from build123d import *

# Parameters (mm, degrees)
F1_DEPTH = 430
F3_DEPTH = 60.001
F4_R     = 4.5
F5_DEPTH = 60.001


with BuildPart() as f1:
    # F0 (on Front) → F1 (new body)
    with BuildSketch(Plane.XZ):
        Polygon((60, 0), (0, 0), (0, -60), (2.5, -60), (2.5, -2.5), (60, -2.5), align=None)
    extrude(amount=F1_DEPTH)

    # F2 (on face) → F3 (cut, through all)
    with BuildSketch(Plane(origin=(0, 0, 0), x_dir=(0, -1, 0), z_dir=(-1, 0, 0))):
        Polygon((0, 0), (0, -60), (60, -60), align=None)
        Polygon((370, -60), (430, -60), (430, 0), align=None)
    extrude(amount=-F3_DEPTH, mode=Mode.SUBTRACT)

    # F4 (on face) → F5 (cut, through all)
    with BuildSketch(Plane.XY):
        with Locations((30, -90)):
            Circle(F4_R)
        with Locations((30, -190)):
            Circle(F4_R)
        with Locations((30, -330)):
            Circle(F4_R)
        with Locations((30, -400)):
            Circle(F4_R)
    extrude(amount=-F5_DEPTH, mode=Mode.SUBTRACT)


solid = f1.part
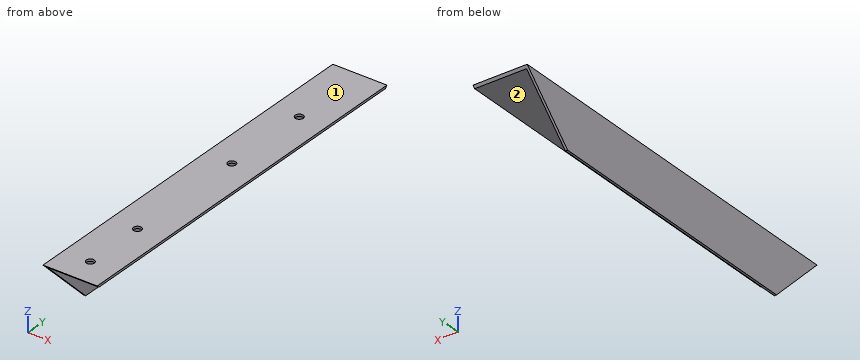
Here's how the part is built. I have some questions about the finished solid (model axes, mm). Face numbers are marked on the shaded views. A direction names the side the tool comes from. Round coordinates to 2 decimals unless told otherwise and drop trailing zeros. Loops run counter-clockwise (first coordinate to the right, second up) from the corner with the lowest first, then second, coordinate; pieces in that order, holes last. Notation, with made-up numbers: M 48.25,-25.75 L 72.25,-25.75 A27 cw 72.25,-1.75 Z; hole C 79.5,-7.5 d3. An arc over 180 degrees is marked long. Write each question's results on one line, items separated by ' | '. Start each with the question number.
(1) I want a section at A-A (y = -330). Please give me the cut outline in (x, z).
(2) On a 3-axis mill with a long thin cutter (end or side, diameter ignored), from which of +Z, -Z, +X, -X, +Y, -Y can I reach the whole of each face in a straight line? I mean the marked faces 1 and 2. Say none if no direction works.
(3) I want a section at C-C (y = -400). Please give me the cut outline in (x, z), then the cut area to 3 significant figures.
(4) I want a section at B-B (x = 30). Please give me the cut outline in (y, z).
(5) If I drill on probe 1 along X at (y, z) = (-330, -1.75); probe 2 along Y at (x, z) = (30, -1.9); probe 3 along Y at (x, z) = (30, -1.45), over which ranges is the centre line in solid material (lowest first)? Write a range as from..to.
(6) Will these pins go through, and if not, where does the flat tip stop? P1, Ø17.5, axis at y = -248, z = -25.5, coming from the +X side; P2, Ø5, axis at x = 8, y = -204, coming from the -Z side.
(7) I want a section at D-D (z = -47.5). Please give me the cut outline in (x, y).
Solved:
1) outline: M 0,-60 L 2.5,-60 L 2.5,-2.5 L 25.5,-2.5 L 25.5,0 L 0,0 Z; M 34.5,-2.5 L 60,-2.5 L 60,0 L 34.5,0 Z
2) face 1: +Z, +X, -X, +Y, -Y | face 2: -Z, +X, +Y, -Y
3) outline: M 0,-30 L 2.5,-30 L 2.5,-2.5 L 25.5,-2.5 L 25.5,0 L 0,0 Z; M 34.5,-2.5 L 60,-2.5 L 60,0 L 34.5,0 Z | area: 196 mm²
4) outline: M -430,0 L -427.5,-2.5 L -404.5,-2.5 L -404.5,0 Z; M -395.5,-2.5 L -334.5,-2.5 L -334.5,0 L -395.5,0 Z; M -325.5,-2.5 L -194.5,-2.5 L -194.5,0 L -325.5,0 Z; M -185.5,-2.5 L -94.5,-2.5 L -94.5,0 L -185.5,0 Z; M -85.5,-2.5 L -2.5,-2.5 L 0,0 L -85.5,0 Z
5) probe 1: x = 0..25.5, 34.5..60 | probe 2: y = -428.1..-404.5, -395.5..-334.5, -325.5..-194.5, -185.5..-94.5, -85.5..-1.9 | probe 3: y = -428.55..-404.5, -395.5..-334.5, -325.5..-194.5, -185.5..-94.5, -85.5..-1.45
6) P1: stops at x = 2.5 | P2: stops at z = -2.5
7) outline: M 0,-382.5 L 2.5,-382.5 L 2.5,-47.5 L 0,-47.5 Z
